```python
from build123d import *

# Parameters (mm, degrees)
F0_W        = 19.05
F0_H        = 6.35
F0_W_2      = 6.35
F0_H_2      = 31.75
F1_DEPTH    = 50.8
F3_DEPTH    = 38.101
F4_R        = 6.35
F5_T1_DEPTH = 68.1131376889


# Not quite as in the source:
# - a fillet or chamfer that OpenCascade refuses, or shapes differently, is made with other operations: its cross-section is extruded or revolved along the edge and cut away or added


with BuildPart() as f1:
    # F0 (on Right) → F1 (new body)
    with BuildSketch(Plane.YZ):
        with Locations((-15.875, 47.625)):
            Rectangle(F0_W, F0_H)
        with Locations((-3.175, 47.625)):
            Rectangle(F0_W_2, F0_H)
        with Locations((-3.175, 28.575)):
            Rectangle(F0_W_2, F0_H_2)
        with BuildLine():
            Line((0, 50.8), (0, 44.45))
            Line((0, 44.45), (4.7625, 44.45))
            ThreePointArc((4.7625, 44.45), (0.8082593776, 28.8201935432), (1.0656091525, 12.7))
            Line((1.0656091525, 12.7), (4.0578971116, 12.7))
            ThreePointArc((4.0578971116, 12.7), (4.3300087855, 32.3527315264), (11.1125, 50.8))
            Line((11.1125, 50.8), (0, 50.8))
        make_face()
    extrude(amount=F1_DEPTH)

    # F2 (on face) → F3 (cut, through all)
    with BuildSketch(Plane.XY.offset(50.8)):
        Polygon((2.3061167124, -15.875), (3.175, -15.875), (4.0438832876, -15.875), (4.0438832876, -15.37335), (3.175, -14.8717), (2.3061167124, -15.37335), align=None)
        Polygon((4.0438832876, -15.875), (3.175, -15.875), (2.3061167124, -15.875), (2.3061167124, -16.37665), (3.175, -16.8783), (4.0438832876, -16.37665), align=None)
        with BuildLine():
            ThreePointArc((47.498, -15.875), (40.64, -9.017), (33.782, -15.875))
            Line((33.782, -15.875), (40.64, -15.875))
            Line((40.64, -15.875), (47.498, -15.875))
        make_face()
        with BuildLine():
            Line((40.64, -15.875), (33.782, -15.875))
            ThreePointArc((33.782, -15.875), (40.64, -22.733), (47.498, -15.875))
            Line((47.498, -15.875), (40.64, -15.875))
        make_face()
        Polygon((24.9555, -14.701824253), (24.9555, -15.875), (26.9875, -15.875), (29.0195, -15.875), (29.0195, -14.701824253), (26.9875, -13.528648506), align=None)
        Polygon((26.9875, -15.875), (24.9555, -15.875), (24.9555, -17.048175747), (26.9875, -18.221351494), (29.0195, -17.048175747), (29.0195, -15.875), align=None)
        Polygon((18.3259538773, -14.9987), (18.3259538773, -15.875), (19.84375, -15.875), (21.3615461227, -15.875), (21.3615461227, -14.9987), (19.84375, -14.1224), align=None)
        Polygon((19.84375, -15.875), (18.3259538773, -15.875), (18.3259538773, -16.7513), (19.84375, -17.6276), (21.3615461227, -16.7513), (21.3615461227, -15.875), align=None)
        Polygon((12.9676772846, -15.113), (12.9676772846, -15.875), (14.2875, -15.875), (15.6073227154, -15.875), (15.6073227154, -15.113), (14.2875, -14.351), align=None)
        Polygon((14.2875, -15.875), (12.9676772846, -15.875), (12.9676772846, -16.637), (14.2875, -17.399), (15.6073227154, -16.637), (15.6073227154, -15.875), align=None)
        Polygon((7.6313977372, -15.24), (7.6313977372, -15.875), (8.73125, -15.875), (9.8311022628, -15.875), (9.8311022628, -15.24), (8.73125, -14.605), align=None)
        Polygon((8.73125, -15.875), (7.6313977372, -15.875), (7.6313977372, -16.51), (8.73125, -17.145), (9.8311022628, -16.51), (9.8311022628, -15.875), align=None)
    extrude(amount=-F3_DEPTH, mode=Mode.SUBTRACT)

    # F4
    f4_edges = [f1.edges().sort_by_distance(p)[0] for p in [
        (25.4, 11.1125, 50.8),
    ]]
    fillet(f4_edges, radius=F4_R)

    # F5: chamfer of 3.175 on 1 edges, made by hand

    # F5_s2 → F5_t1 (cut)
    with BuildSketch(Plane.YZ.offset(-8.6565688444)):
        with BuildLine():
            Line((4.422273237, 12.6144658264), (0.5675477916, 16.1266199594))
            Line((0.5675477916, 16.1266199594), (0.5043218231, 16.1207270056))
            ThreePointArc((0.5043218231, 16.1207270056), (0.7717830499, 14.4079265456), (1.0028018544, 12.690646214))
            Line((1.0028018544, 12.690646214), (1.0656091525, 12.6365))
            ThreePointArc((1.0656091525, 12.6365), (2.7439411948, 12.6365), (4.422273237, 12.5509658264))
            Line((4.422273237, 12.5509658264), (4.422273237, 12.6144658264))
        make_face()
    extrude(amount=F5_T1_DEPTH, mode=Mode.SUBTRACT)


solid = f1.part
```
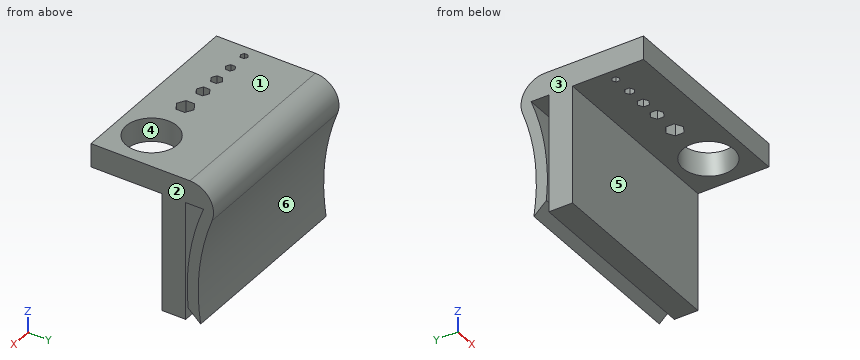
CAD build for the part. Positions are in the model's coordinates, mm. Face numbers are marked on the shaded views. A direction names the side the tool comes from. Coordinates: 2 decimals unless noted, no trailing zeros. Loops run counter-clockwise (first coordinate to the right, second up) from the corner with the lowest first, then second, coordinate; pieces in that order, holes last. Notation, with made-up numbers: (55, 89) - (96, 89) arc R28 cw to (96, 110) - close; hole circle Ø8 at (75, -17.75). An arc over 180 degrees is marked (long way). Return JSON: item names as keys, results as strings.
1. Mould opens along X. For the marked faces 1, 2, 3 and 4 say: released by +X, released by -X, zero draft, split by the parting line, or undercut.
Result:
{"face 1": "zero draft", "face 2": "released by +X", "face 3": "released by -X", "face 4": "undercut"}
2. Probe L1, parallel to X at y = -14, z = 46.5; L2, parallel to X at y = -13, z = 47; L3, parallel to Z at x = 44, y = -8. List the from-to ranges inside material, lowest first. Write a range as from..to.
Result:
{"L1": "x = 0..26.17, 27.8..34.04, 47.24..50.8", "L2": "x = 0..34.41, 46.87..50.8", "L3": "z = 44.45..50.8"}
3. Band-saw the part on C-C (y = -12.5). Give the cut face in (x, z), and give its area (3 significant figures).
Result:
{"outline": "(0, 44.45) - (34.67, 44.45) - (34.67, 50.8) - (0, 50.8) - close; (46.61, 44.45) - (50.8, 44.45) - (50.8, 50.8) - (46.61, 50.8) - close", "area": "247 mm2"}
4. Band-saw the part on B-B (z = 26.5). Give the cut face in (x, y).
Result:
{"outline": "(0, -6.35) - (50.8, -6.35) - (50.8, 0) - (0, 0) - close; (0, 0.58) - (50.8, 0.58) - (50.8, 3.55) - (0, 3.55) - close"}
5. Drop flat-ended pins along their axis: pin 1 (2.5 mm diameter, centred on x = 23, y = 2.5, fed in from -Z); pin 2 (3 mm diameter, centred on x = 22.5, y = -13.5, fed in from -Z); pin 3 (1 mm diameter, centred on x = 12, z = 39.5, fed in from +Y). Give the stop position or say it passes through.
Result:
{"pin 1": "stops at z = 13.23", "pin 2": "stops at z = 44.45", "pin 3": "stops at y = 6.29"}
6. 3-axis set-ups, long thin cutter, end or side, ignore diameter. For the marked faces 5 and 6: which of +Z, -Z, +X, -X, +Y, -Y reach the whole face in a straight line?
Result:
{"face 5": "-Z, +X, -X, -Y", "face 6": "+X, -X, +Y"}
7. Band-saw the part on A-A (x = 40.64). Give the cut face in (y, z).
Result:
{"outline": "(-25.4, 44.45) - (-22.73, 44.45) - (-22.73, 50.8) - (-25.4, 50.8) - close; (-9.02, 44.45) - (-6.35, 44.45) - (-6.35, 12.7) - (0, 12.7) - (0, 44.45) - (4.76, 44.45) arc R61.3 ccw to (0.66, 16.04) - (4.01, 12.99) arc R58.34 cw to (7.07, 42.22) arc R6.35 ccw to (1.13, 50.8) - (-9.02, 50.8) - close"}
